Build history of the part. All positions in model axes, mm. Face numbers are marked on the shaded views. A direction names the side the tool comes from. Round coordinates to 2 decimals unless told otherwise and drop trailing zeros. Order: outer loops, then holes, each group sorted by start corner. A loop starts at its lowest first (then second) coordinate and runs counter-clockwise, first axis right, second up. Notation, with made-up numbers: (33.25, 13.5) -> (77.25, 13.5) arc R11 ccw to (77.25, 26.5) -> close; hole circle Ø9 at (0, 35.25). An arc over 180 degrees is marked (long way). Answer as a JSON object with one key per item and string values.
Autodesk Inventor part; units mm, degrees
ref_plane "Plano de trabajo1" through (0, 0, -65) normal (0, 0, 1) x (1, 0, 0)
ref_plane "Plano de trabajo2" through (0, 0, -65) normal (0, 0, 1) x (1, 0, 0)
ref_plane "Plano de trabajo3" through (0, 0, -65) normal (0, 0, 1) x (1, 0, 0)
sketch "Boceto1" plane through (0, 0, 0) normal (0, 1, 0) x (-1, 0, 0)
  line L0 (197.3419, -130) -> (35, -130)
  line L1 (5, -32.5) -> (30, -32.5)
  line L2 (30, -32.5) -> (30, -97.5)
  line L3 (30, -97.5) -> (5, -97.5)
  line L4 (30, -5) -> (30, -32.5)
  line L5 (30, -97.5) -> (30, -125)
  line L6 (0, -37.5) -> (0, -92.5)
  arc A0 (5, -32.5) -> (0, -37.5) centre (5, -37.5) ccw
  arc A1 (0, -92.5) -> (5, -97.5) centre (5, -92.5) ccw
  line L7 (35, 0) -> (40, 0) construction
  line L8 (40, 0) -> (40, -130) construction
  line L9 (40, -130) -> (70, -130)
  line L10 (70, -130) -> (70, -75)
  line L11 (70, -75) -> (40, -75)
  line L12 (40, -75) -> (40, -130)
  line L13 (40, 0) -> (70, 0)
  line L14 (70, 0) -> (70, -55)
  line L15 (70, -55) -> (40, -55)
  line L16 (40, -55) -> (40, 0)
  arc A2 (30, -125) -> (35, -130) centre (35, -125) ccw
  arc A3 (35, 0) -> (30, -5) centre (35, -5) ccw
  line L17 (70, 0) -> (70, -5) construction
  line L18 (70, -130) -> (70, -125) construction
  line L19 (70, -125) -> (195, -125)
  line L20 (70, -5) -> (195, -5)
  line L21 (195, -5) -> (220, -5) construction
  line L22 (220, -5) -> (220, -125) construction
  line L23 (220, -125) -> (195, -125) construction
  line L24 (0, -65) -> (285, -65) construction
  line L25 (220, -65) -> (220, -95) construction
  line L26 (220, -65) -> (220, -35) construction
  line L27 (220, -35) -> (255, -35) construction
  line L28 (255, -35) -> (255, -95) construction
  line L29 (255, -95) -> (220, -95) construction
  line L30 (195, -5) -> (220, -35)
  line L31 (195, -125) -> (220, -95)
  line L32 (220, -95) -> (255, -95)
  line L33 (220, -35) -> (255, -35)
  line L34 (255, -35) -> (255, -95)
  line L35 (207.5, -110) -> (211.3411, -113.2009) construction
  line L36 (197.3419, -130) -> (226.5085, -95)
  line L37 (197.3419, 0) -> (226.5085, -35)
  line L38 (70, 0) -> (197.3419, 0)
  line L39 (35, 0) -> (40, 0)
  line L40 (255, -95) -> (258, -95)
  line L41 (258, -95) -> (258, -35)
  line L42 (258, -35) -> (255, -35)
  line L43 (255, -35) -> (255, -95)
  point P0 (0, 0)
  point P1 (30, -130)
  dimension "d5" = 5
  dimension "d7" = 30
  dimension "d8" = 55
  dimension "d9" = 55
  dimension "d10" = 5
  dimension "d11" = 5
  dimension "d12" = 125
  dimension "d13" = 25
  dimension "d14" = 30
  dimension "d15" = 30
  dimension "d16" = 35
  dimension "d17" = 5
  dimension "d62" = 3
extrude "Extrusión1" add sketch "Boceto1" along normal blind 40 contours L0 L10 L19 L31 L32 L36 | L33 L30 L20 L14 L38 L37
extrude "Extrusión2" add sketch "Boceto1" along normal blind 5 contours L32 L31 L19 L10 L11 L12 L0 A2 L5 L2 L4 A3 L39 L16 L15 L14 L20 L30 L33 L34 | L34 L42 L41 L40 | L3 A1 L6 A0 L1 L2
extrude "Extrusión3" add sketch "Boceto1" along normal blind 20 contours L0 L12 L11 L10 | L14 L15 L16 L13
fillet "Empalme1" radius 5 2 edges at (-197.3419, 20, 0) (-197.3419, 20, -130)
ref_plane "Plano de trabajo1" through (0, 0, -65) normal (0, 0, 1) x (1, 0, 0)
sketch "Boceto2" plane through (0, 0, -65) normal (0, 0, 1) x (1, 0, 0)
  line L0 (-40, 20) -> (-70, 20) construction
  line L1 (-70, 20) -> (-68, 20) construction
  line L2 (-40, 5) -> (-40, 20) construction
  line L3 (-40, 20) -> (-42, 20) construction
  arc A0 (-68, 20) -> (-42, 20) centre (-55, 18.1333) ccw
  line L4 (-68, 20) -> (-68, 21.6532)
  line L5 (-68, 21.6532) -> (-42, 21.6532)
  line L6 (-42, 21.6532) -> (-42, 20)
  point P0 (0, 0)
  dimension "d26" = 2
  dimension "d27" = 2
extrude "Extrusión4" cut sketch "Boceto2" along normal mid plane 126
sketch "Boceto3" plane through (0, 0, -65) normal (0, 0, 1) x (1, 0, 0)
  line L0 (-68, 20) -> (-42, 20) construction
  line L1 (-55, 20) -> (-59, 20) construction
  line L2 (-55, 20) -> (-51, 20) construction
  line L3 (-55, 20) -> (-55, 16.5) construction
  arc A0 (-59, 20) -> (-51, 20) centre (-55, 20.5357) ccw
  arc A1 (-51, 20) -> (-59, 20) centre (-55, 15.3068) ccw
  point P0 (0, 0)
  dimension "d30" = 4
  dimension "d33" = 3.5
extrude "Extrusión5" cut sketch "Boceto3" along normal through all both and the other way through all
sketch "Boceto4" plane through (0, 0, -65) normal (0, 0, 1) x (1, 0, 0)
  arc A0 (-59, 20) -> (-51, 20) centre (-55, 20.5357) ccw construction
  line L0 (-55, 16.5) -> (-55, 13.5) construction
  circle A1 centre (-55, 13.5) radius 1.5
  point P0 (0, 0)
  dimension "d36" = 3
  dimension "d37" = 3
extrude "Extrusión6" cut sketch "Boceto4" along normal through all both and the other way through all
sketch "Boceto5" plane through (0, 5, 0) normal (0, 1, 0) x (1, 0, 0)
  line L0 (-30, 97.5) -> (-30, 125) construction
  line L1 (-30, 32.5) -> (-30, 97.5) construction
  line L2 (0, 37.5) -> (0, 92.5) construction
  line L3 (0, 65) -> (-30, 65) construction
  line L4 (0, 97.5) -> (-15, 97.5) construction
  line L5 (-5, 97.5) -> (-30, 97.5) construction
  line L6 (-15, 97.5) -> (-15, 32.5) construction
  line L7 (-30, 32.5) -> (-5, 32.5) construction
  line L8 (-15, 65) -> (-15, 40) construction
  line L9 (-15, 40) -> (-20, 40) construction
  line L10 (-20, 40) -> (-22, 40) construction
  circle A0 centre (-22, 40) radius 2
  circle A1 centre (-8, 40) radius 2
  circle A2 centre (-22, 90) radius 2
  circle A3 centre (-8, 90) radius 2
  point P0 (0, 0)
  dimension "d40" = 15
  dimension "d41" = 25
  dimension "d42" = 5
  dimension "d43" = 2
extrude "Extrusión7" cut sketch "Boceto5" against normal blind 10
sketch "Boceto6" plane through (0, 5, 0) normal (0, 1, 0) x (1, 0, 0)
  line L0 (-70, 55) -> (-70, 5) construction
  line L1 (-70, 5) -> (-70, 10) construction
  line L2 (-70, 10) -> (-75, 10) construction
  line L3 (-75, 10) -> (-75, 5) construction
  line L4 (-75, 5) -> (-70, 10) construction
  line L5 (-75, 10) -> (-70, 5) construction
  circle A0 centre (-72.5, 7.5) radius 2
  arc A1 (-70, 10) -> (-75, 5) centre (-72.5, 7.5) ccw
  line L6 (-70, 0) -> (-70, 5)
  line L7 (-70, 10) -> (-70, 5)
  line L8 (-70, 5) -> (-75, 5)
  line L9 (0, 37.5) -> (0, 92.5) construction
  line L10 (0, 65) -> (-255, 65) construction
  line L11 (-255, 95) -> (-255, 35) construction
  line L12 (0, 65) -> (-127.5, 65) construction
  line L13 (-127.5, 65) -> (-127.5, 0) construction
  line L14 (-195, 0) -> (-35, 0) construction
  line L15 (-70, 125) -> (-70, 120) construction
  circle A2 centre (-72.5, 122.5) radius 2
  arc A3 (-75, 125) -> (-70, 120) centre (-72.5, 122.5) ccw
  line L16 (-70, 120) -> (-70, 125)
  line L17 (-70, 125) -> (-75, 125)
  line L18 (-195, 5) -> (-220, 35) construction
  line L19 (-195, 125) -> (-70, 125) construction
  line L20 (-195, 5) -> (-195, 125) construction
  line L21 (-70, 65) -> (-132.5, 65) construction
  line L22 (-132.5, 65) -> (-132.5, 130) construction
  line L23 (-35, 130) -> (-195, 130) construction
  circle A4 centre (-192.5, 7.5) radius 2
  arc A5 (-190, 5) -> (-195, 10) centre (-192.5, 7.5) ccw
  line L24 (-195, 10) -> (-195, 5)
  line L25 (-195, 5) -> (-190, 5)
  arc A6 (-195, 120) -> (-190, 125) centre (-192.5, 122.5) ccw
  circle A7 centre (-192.5, 122.5) radius 2
  line L26 (-195, 125) -> (-190, 125)
  line L27 (-195, 120) -> (-195, 125)
  arc A8 (-195, 125) -> (-192.5, 118.9645) centre (-192.5, 122.5) ccw
  line L28 (-190, 125) -> (-195, 125)
  arc A9 (-192.5, 11.0355) -> (-195, 5) centre (-192.5, 7.5) ccw
  point P0 (0, 0)
  point P1 (-195, 120)
  dimension "d47" = 5
  dimension "d48" = 4
  dimension "d49" = 127.5
  dimension "d50" = 62.5
extrude "Extrusión8" add sketch "Boceto6" along normal blind 35
extrude "Extrusión9" cut sketch "Boceto6" against normal blind 35 contours A0 | A2 | A4 | A7
sketch "Boceto7" plane through (0, 5, 0) normal (0, 1, 0) x (1, 0, 0)
  line L0 (-255, 35) -> (-226.5085, 35) construction
  line L1 (-198.8411, 128.2009) -> (-226.5085, 95) construction
  line L2 (-226.5085, 35) -> (-226.5085, 95) construction
  line L3 (-226.5085, 65) -> (-255, 65) construction
  line L4 (-255, 95) -> (-255, 35) construction
  line L5 (-226.5085, 95) -> (-255, 95) construction
  line L6 (-240.7543, 95) -> (-240.7543, 35) construction
  line L7 (-226.5085, 35) -> (-229.5085, 35) construction
  circle A0 centre (-252, 40) radius 2
  circle A1 centre (-252, 90) radius 2
  line L8 (-226.5085, 35) -> (-226.5085, 40) construction
  line L9 (-226.5085, 40) -> (-232.0085, 40) construction
  circle A2 centre (-232.0085, 40) radius 2
  circle A3 centre (-232.0085, 90) radius 2
  point P0 (0, 0)
  dimension "d64" = 5.5
  dimension "d65" = 4
extrude "Extrusión10" cut sketch "Boceto7" against normal blind 35
ref_plane "Plano de trabajo2" through (0, 0, -65) normal (0, 0, 1) x (1, 0, 0)
ref_plane "Plano de trabajo3" through (0, 0, -65) normal (0, 0, 1) x (1, 0, 0)
sketch "Boceto9" plane through (0, 0, -65) normal (0, 0, 1) x (1, 0, 0)
  line L0 (-226.5085, 5) -> (-226.5085, 40) construction
  line L1 (-226.5085, 22.5) -> (-226.5085, 27)
  line L2 (-226.5085, 27) -> (-204.8867, 27)
  line L3 (-204.8867, 27) -> (-204.8867, 13)
  line L4 (-204.8867, 13) -> (-226.5085, 13)
  line L5 (-226.5085, 13) -> (-226.5085, 27)
  point P0 (0, 0)
  dimension "d79" = 4.5
  dimension "d80" = 14
extrude "Extrusión12" cut sketch "Boceto9" along normal through all both and the other way through all
fillet "Empalme2" radius 2 8 edges at (-204.8867, 20, -16.864) (-204.8867, 20, -9.0538) (-204.8867, 20, -120.9462) (-204.8867, 20, -113.136) (-220, 33.5, -35) (-226.5085, 33.5, -35) (-226.5085, 33.5, -95) (-220, 33.5, -95)
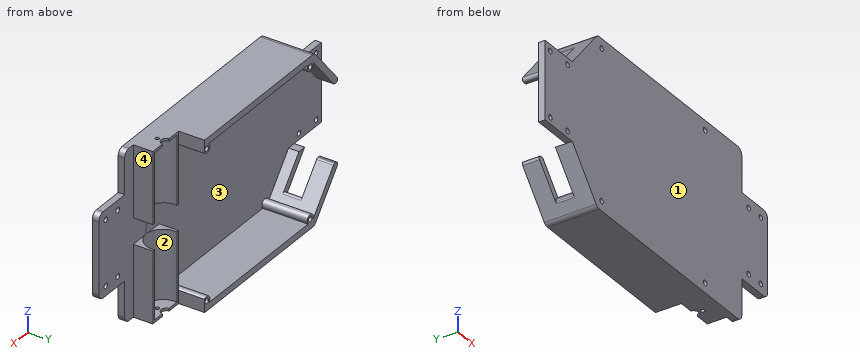
1) Cut at B-B, the plane z = -27. Give the cut face in (x, y), plus the area to 3 significant figures.
Checked values:
{"outline": "(-219.84, 0) -> (-30, 0) -> (-30, 5) -> (-40, 5) -> (-40, 20) -> (-42, 20) arc R13.13 cw (long way) to (-68, 20) -> (-70, 20) -> (-70, 5) -> (-213.33, 5) -> (-213.33, 13) -> (-219.84, 13) -> close; (-219.84, 27) -> (-213.33, 27) -> (-213.33, 40) -> (-219.84, 40) -> close", "area": "1,220 mm²"}
2) Cut at D-D, the plane z = -83.5. Give the cut face in (x, y).
Checked values:
{"outline": "(-258, 0) -> (0, 0) -> (0, 5) -> (-40, 5) -> (-40, 20) -> (-42, 20) arc R13.13 cw (long way) to (-68, 20) -> (-70, 20) -> (-70, 5) -> (-258, 5) -> close"}
3) Probe L1, parallel to Z at x = -72.5, y = 24.5; L2, parallel to X at y = 2, z = -40; L3, parallel to Z at x = -22, y = 2.95. List the from-to ranges inside material, lowest first. Write a range as from..to.
Checked values:
{"L1": "z = -130..-124.5, -120.5..-118.96, -11.04..-9.5, -5.5..0", "L2": "x = -258..-254, -250..-234.01, -230.01..-24, -20..-10, -6..0", "L3": "z = -97.5..-92, -88..-42, -38..-32.5"}
4) Cut at C-C, the plane x = -119.5. Give the cut face in (y, z).
Checked values:
{"outline": "(0, -130) -> (40, -130) -> (40, -125) -> (5, -125) -> (5, -5) -> (40, -5) -> (40, 0) -> (0, 0) -> close"}
5) Flat gauge pins, fed straight in: pin 1 Ø5.5 at (x, y) = (-248, 1.5) entering from +Z; pin 2 Ø2.5 at (x, z) = (-192.5, -7.5) entering from +Y; pin 3 Ø3 at (y, z) = (18, -22.5) entering from -X; pin 4 Ø5.5 at (x, z) = (-63.5, -97) entering from +Y. Where does each tip first touch, or does it go through?
Checked values:
{"pin 1": "stops at z = -35", "pin 2": "passes through", "pin 3": "stops at x = -70", "pin 4": "stops at y = 11.36"}
6) Which spindle directions (+Z, -Z, +X, -X, +Y, -Y) get a long thin tool onto all of the face, cutting with end or side? Do the marked faces 1, 2, 3 and 4. Say none if no direction does.
Checked values:
{"face 1": "+Z, -Z, +X, -X, -Y", "face 2": "none", "face 3": "+Y", "face 4": "+Z, -Z, +X, +Y"}
7) Cut at A-A, the plane y = 31.5. Give the cut face in (x, z), plus the area to 3 significant figures.
Checked values:
{"outline": "(-223.77, -98.28) -> (-198.84, -128.2) arc R5 ccw to (-195, -130) -> (-70, -130) -> (-70, -120) arc R3.54 ccw to (-75, -125) -> (-190, -125) arc R3.54 ccw to (-195, -120) arc R3.54 ccw to (-195.41, -124.51) -> (-219.4, -95.72) arc R2 ccw to (-220.94, -95) -> (-222.24, -95) arc R2 ccw to start; (-223.77, -31.72) arc R2 ccw to (-222.24, -35) -> (-220.94, -35) arc R2 ccw to (-219.4, -34.28) -> (-195.41, -5.49) arc R3.54 ccw to (-195, -10) arc R3.54 ccw to (-190, -5) -> (-75, -5) arc R3.54 ccw to (-70, -10) -> (-70, 0) -> (-195, 0) arc R5 ccw to (-198.84, -1.8) -> close; hole circle Ø4 at (-192.5, -122.5); hole circle Ø4 at (-192.5, -7.5); hole circle Ø4 at (-72.5, -122.5); hole circle Ø4 at (-72.5, -7.5)", "area": "1,760 mm²"}
